Geometry check sheet. Reference: drawing and pictorial views, mm from the part's lowest x, y, z. Coordinates: 2 decimals unless noted, no trailing zeros. Write each loop counter-clockwise with the first axis right and the second up, starting at its lowest first coordinate (ties: lowest second). Pieces come first, ordered by that corner, then holes. Notation, with made-up numbers: (86, -6.5) -> (140, -6.5) arc R16 ccw to (140, 2.5) -> close; hole circle Ø2 at (48, 31.5). An arc over 180 degrees is marked (long way). Use a Markdown table: item, result. Add a question column.
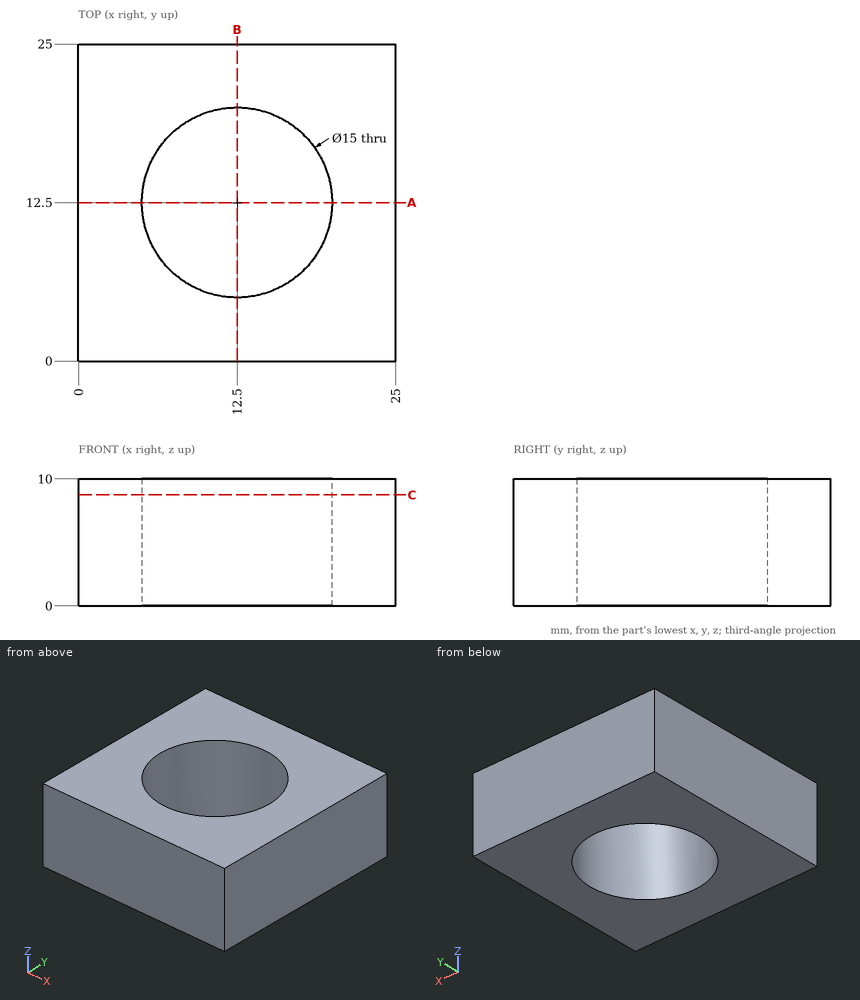
1) Cross-section at A-A on y = 12.5. Record the boundary of the cut face in (x, z), then the cut area to 3 significant figures.
2) Cross-section at C-C on z = 8.75. Record the boundary of the cut face in (x, y), then the cut area to 3 significant figures.
3) Thickness scan on L1, parallel to Y at x = 12.5, z = 7; L2, parallel to Y at x = 9.75, z = 4.75. Record the ranges inside material, lowest first.
4) Gauge pin test, flat ends, axial feed: pin 1 (3 mm diameter, centred on x = 20, z = 5.5, fed in from -Y); pin 2 (5 mm diameter, centred on x = 9.5, y = 11.5, fed in from -Z). Record the tip position at first contact, or that the pin passes through.
Returned:
| question | item | result |
|---|---|---|
| 1 | outline | (0, 0) -> (5, 0) -> (5, 10) -> (0, 10) -> close; (20, 0) -> (25, 0) -> (25, 10) -> (20, 10) -> close |
| 1 | area | 100 mm² |
| 2 | outline | (0, 0) -> (25, 0) -> (25, 25) -> (0, 25) -> close; hole circle Ø15 at (12.5, 12.5) |
| 2 | area | 448 mm² |
| 3 | L1 | y = 0 to 5, 20 to 25 |
| 3 | L2 | y = 0 to 5.52, 19.48 to 25 |
| 4 | pin 1 | stops at y = 0 |
| 4 | pin 2 | passes through |
